Drawing for the job (mm, zero at the part's lowest x, y, z). Round coordinates to 2 decimals unless told otherwise and drop trailing zeros. Loops run counter-clockwise (first coordinate to the right, second up) from the corner with the lowest first, then second, coordinate; pieces in that order, holes last. Notation, with made-up numbers: M -26,-39.75 L 4,-39.75 A9 cw 4,-32.75 Z; hole C -15.75,46.25 d9. An arc over 180 degrees is marked long. Use a Markdown table: item, result. Add a question column.
Q1. Cut at A-A (x = 125). Give the cut face in (y, z) (3 decimals), plus the area to 3 significant figures.
Q2. Probe line 1 (Y direction, x = 125, z = 2.1); line 2 (Y direction, x = 59.5, z = 1.5); line 3 (X direction, y = 57.5, z = 2.1). List the from-to ranges inside material, lowest first. Write a range as from..to.
Q3. Cut at B-B (z = 1.85). Give the cut face in (x, y).
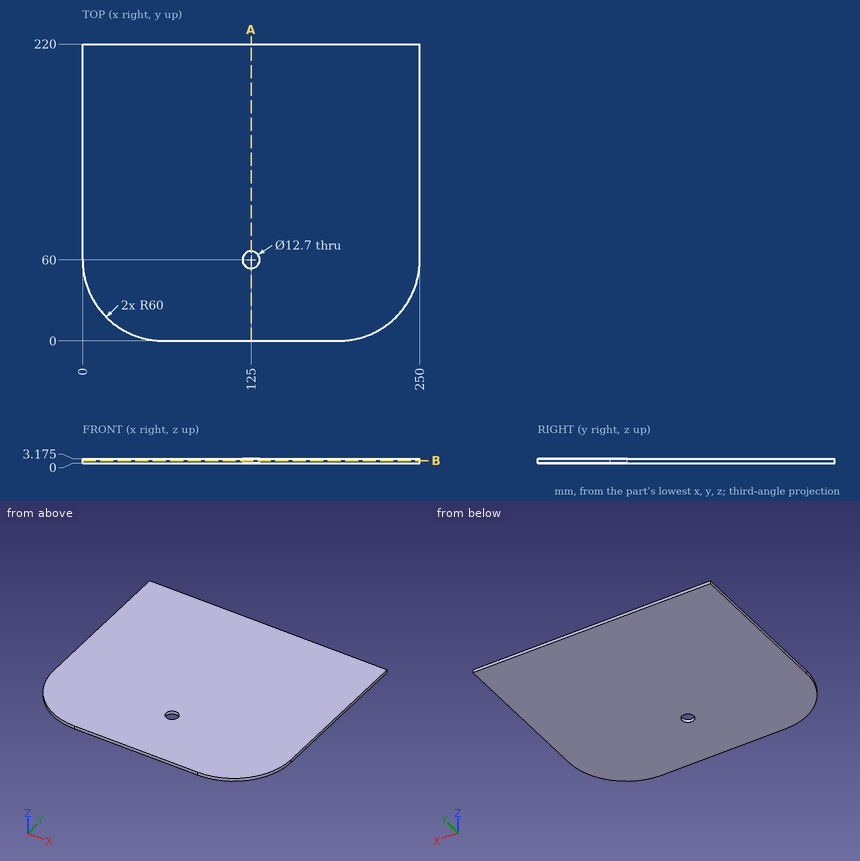
Checked values:
| question | item | result |
|---|---|---|
| 1 | outline | M 0,0 L 53.65,0 L 53.65,3.175 L 0,3.175 Z; M 66.35,0 L 220,0 L 220,3.175 L 66.35,3.175 Z |
| 1 | area | 658 mm^2 |
| 2 | line 1 | y = 0..53.65, 66.35..220 |
| 2 | line 2 | y = 0..220 |
| 2 | line 3 | x = 0.05..119.16, 130.84..249.95 |
| 3 | outline | M 0,60 A60 ccw 60,0 L 190,0 A60 ccw 250,60 L 250,220 L 0,220 Z; hole C 125,60 d12.7 |
